Geometry: final body of the model. Coordinates: model frame, mm. Face numbers are marked on the shaded views. Round coordinates to 2 decimals unless told otherwise and drop trailing zeros. Loops run counter-clockwise (first coordinate to the right, second up) from the corner with the lowest first, then second, coordinate; pieces in that order, holes last. Notation, with made-up numbers: M 12.25,-4.75 L 49.25,-4.75 A20 ccw 49.25,16.25 Z; hole C 29.5,-14 d8. An arc over 180 degrees is marked long. Answer as a JSON object with one key per item and string values.
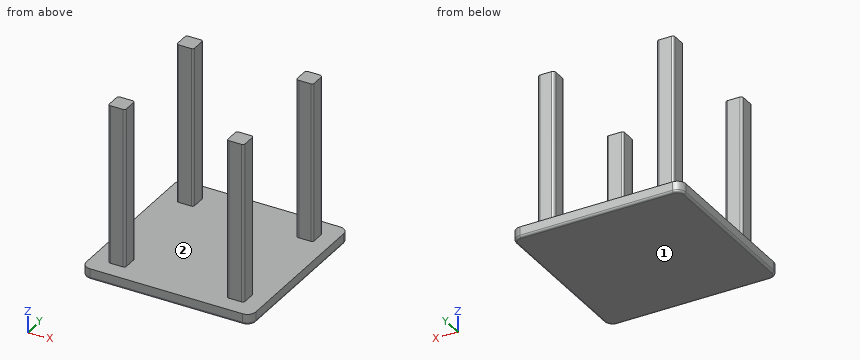
```python
from build123d import *

# Parameters (mm, degrees)
F1_DEPTH = 25
F6_DEPTH = 375
F7_R     = 5


with BuildPart() as f1:
    # F0 (on Top) → F1 (new body)
    with BuildSketch(Plane.XY):
        with BuildLine():
            Line((184.353015, 213.828545), (-175.646985, 213.828545))
            ThreePointArc((-175.646985, 213.828545), (-189.789121, 207.97068), (-195.646985, 193.828545))
            Line((-195.646985, 193.828545), (-195.646985, -166.171455))
            ThreePointArc((-195.646985, -166.171455), (-189.789121, -180.313591), (-175.646985, -186.171455))
            Line((-175.646985, -186.171455), (184.353015, -186.171455))
            ThreePointArc((184.353015, -186.171455), (198.49515, -180.313591), (204.353015, -166.171455))
            Line((204.353015, -166.171455), (204.353015, 193.828545))
            ThreePointArc((204.353015, 193.828545), (198.49515, 207.97068), (184.353015, 213.828545))
        make_face()
    extrude(amount=F1_DEPTH)

    # F2 (on face) + F3 (on face) + F4 (on face) + F5 (on face) → F6 (join)
    with BuildSketch(Plane.XY.offset(25)):
        with BuildLine():
            Line((-120.646985, 173.828545), (-150.646985, 173.828545))
            ThreePointArc((-150.646985, 173.828545), (-154.182519, 172.364079), (-155.646985, 168.828545))
            Line((-155.646985, 168.828545), (-155.646985, 138.828545))
            ThreePointArc((-155.646985, 138.828545), (-154.182519, 135.293011), (-150.646985, 133.828545))
            Line((-150.646985, 133.828545), (-120.646985, 133.828545))
            ThreePointArc((-120.646985, 133.828545), (-117.111451, 135.293011), (-115.646985, 138.828545))
            Line((-115.646985, 138.828545), (-115.646985, 168.828545))
            ThreePointArc((-115.646985, 168.828545), (-117.111451, 172.364079), (-120.646985, 173.828545))
        make_face()
    with BuildSketch(Plane.XY.offset(25)):
        with BuildLine():
            Line((-120.646985, -106.171455), (-150.646985, -106.171455))
            ThreePointArc((-150.646985, -106.171455), (-154.182519, -107.635921), (-155.646985, -111.171455))
            Line((-155.646985, -111.171455), (-155.646985, -141.171455))
            ThreePointArc((-155.646985, -141.171455), (-154.182519, -144.706989), (-150.646985, -146.171455))
            Line((-150.646985, -146.171455), (-120.646985, -146.171455))
            ThreePointArc((-120.646985, -146.171455), (-117.111451, -144.706989), (-115.646985, -141.171455))
            Line((-115.646985, -141.171455), (-115.646985, -111.171455))
            ThreePointArc((-115.646985, -111.171455), (-117.111451, -107.635921), (-120.646985, -106.171455))
        make_face()
    with BuildSketch(Plane.XY.offset(25)):
        with BuildLine():
            Line((159.640082, 173.828545), (132.935292, 173.828545))
            ThreePointArc((132.935292, 173.828545), (128.234725, 171.881506), (126.287687, 167.18094))
            Line((126.287687, 167.18094), (126.287687, 140.476149))
            ThreePointArc((126.287687, 140.476149), (128.234725, 135.775583), (132.935292, 133.828545))
            Line((132.935292, 133.828545), (161.287687, 133.828545))
            ThreePointArc((161.287687, 133.828545), (164.823221, 135.293011), (166.287687, 138.828545))
            Line((166.287687, 138.828545), (166.287687, 167.18094))
            ThreePointArc((166.287687, 167.18094), (164.340649, 171.881506), (159.640082, 173.828545))
        make_face()
    with BuildSketch(Plane.XY.offset(25)):
        with BuildLine():
            Line((159.353015, -106.171455), (129.353015, -106.171455))
            ThreePointArc((129.353015, -106.171455), (125.817481, -107.635921), (124.353015, -111.171455))
            Line((124.353015, -111.171455), (124.353015, -141.171455))
            ThreePointArc((124.353015, -141.171455), (125.817481, -144.706989), (129.353015, -146.171455))
            Line((129.353015, -146.171455), (159.353015, -146.171455))
            ThreePointArc((159.353015, -146.171455), (162.888549, -144.706989), (164.353015, -141.171455))
            Line((164.353015, -141.171455), (164.353015, -111.171455))
            ThreePointArc((164.353015, -111.171455), (162.888549, -107.635921), (159.353015, -106.171455))
        make_face()
    extrude(amount=F6_DEPTH)

    # F7
    f7_edges = [f1.edges().sort_by_distance(p)[0] for p in [
        (4.353015, -186.171455, 0),
    ]]
    fillet(f7_edges, radius=F7_R)


solid = f1.part
```
1) Pull-direction query (X, two-part tool) for the marked faces 1 and 2; classes: +X half, -X half, draft (parallel to the pull), parting line (faces both ways), or undercut.
Geometry results:
{"face 1": "draft", "face 2": "undercut"}
2) Cut plane D-D on y = -7. Return the cut outline in (x, z), and give its area (3 significant figures).
Geometry results:
{"outline": "M -195.65,5 A5 ccw -190.65,0 L 199.35,0 A5 ccw 204.35,5 L 204.35,25 L -195.65,25 Z", "area": "9,990 mm2"}
3) First-contact query: pin 1 (15 mm diameter, centred on y = -125, z = 158.5, fed in from -X); pin 2 (15 mm diameter, centred on y = -128, z = 223.5, fed in from +X); pin 3 (9 mm diameter, centred on x = -136.5, z = 152, fed in from -Y); pin 4 (10 mm diameter, centred on x = -110, z = 158.5, fed in from +Y). Flat tips, straight axial feed; report the tip coordinate or a pass-through.
Geometry results:
{"pin 1": "x = -155.65", "pin 2": "x = 164.35", "pin 3": "y = -146.17", "pin 4": "through"}
4) Line query: probe 1 along Y at (x, z) = (139, 163); probe 2 along X at (y, z) = (146, 103); probe 3 along Z at (x, y) = (127.5, 102). Output: solid intervals per line, ascending.
Geometry results:
{"probe 1": "-146.17 to -106.17, 133.83 to 173.83", "probe 2": "-155.65 to -115.65, 126.29 to 166.29", "probe 3": "0 to 25"}
5) Cut plane A-A on z = 68. Count the separate pieces of the cut face and the enclosed holes in it, and give its area (3 significant figures).
Geometry results:
{"separate pieces": "4", "enclosed holes": "0", "area": "6,300 mm2"}
6) Cut plane B-B on y = -125. Return the cut outline in (x, z).
Geometry results:
{"outline": "M -195.65,5 A5 ccw -190.65,0 L 199.35,0 A5 ccw 204.35,5 L 204.35,25 L 164.35,25 L 164.35,400 L 124.35,400 L 124.35,25 L -115.65,25 L -115.65,400 L -155.65,400 L -155.65,25 L -195.65,25 Z"}
7) Cut plane C-C on x = -129. Return the cut outline in (y, z).
Geometry results:
{"outline": "M -186.17,5 A5 ccw -181.17,0 L 208.83,0 A5 ccw 213.83,5 L 213.83,25 L 173.83,25 L 173.83,400 L 133.83,400 L 133.83,25 L -106.17,25 L -106.17,400 L -146.17,400 L -146.17,25 L -186.17,25 Z"}
